```python
from build123d import *

# Parameters (mm, degrees)
BOSS_EXTRUDE1_DEPTH = 10
BOSS_EXTRUDE2_START = -5
SKETCH1_4_R         = 1.1
BOSS_EXTRUDE2_DEPTH = 5
FILLET1_R           = 3
SKETCH4_W           = 7.2
SKETCH4_H           = 7.2
CUT_EXTRUDE1_DEPTH  = 10
CIRPATTERN1_COUNT   = 3


with BuildPart() as part:
    # Sketch1 → Boss-Extrude1 (new body)
    with BuildSketch(Plane.XY):
        with BuildLine():
            ThreePointArc((-5.777817459, -11.645463727), (-3.344718433, -12.562358799), (-0.777817459, -12.976709907))
            Line((-0.777817459, -12.976709907), (-0.777817459, -0.777817459))
            ThreePointArc((-0.777817459, -0.777817459), (-0.420951776, 1.016267486), (1.1, 0))
            ThreePointArc((1.1, 0), (1.016267486, -0.420951776), (0.777817459, -0.777817459))
            Line((0.777817459, -0.777817459), (0.777817459, -12.976709907))
            ThreePointArc((0.777817459, -12.976709907), (3.344718433, -12.562358799), (5.777817459, -11.645463727))
            ThreePointArc((5.777817459, -11.645463727), (11.047887286, -6.851582774), (13, 0))
            ThreePointArc((13, 0), (-6.851582774, 11.047887286), (-5.777817459, -11.645463727))
        make_face()
        with BuildLine():
            Line((-5.777817459, -20.777817459), (-0.777817459, -20.777817459))
            Line((-0.777817459, -20.777817459), (-0.777817459, -12.976709907))
            ThreePointArc((-0.777817459, -12.976709907), (-3.344718433, -12.562358799), (-5.777817459, -11.645463727))
            Line((-5.777817459, -11.645463727), (-5.777817459, -20.777817459))
        make_face()
        with BuildLine():
            ThreePointArc((5.777817459, -11.645463727), (3.344718433, -12.562358799), (0.777817459, -12.976709907))
            Line((0.777817459, -12.976709907), (0.777817459, -20.777817459))
            Line((0.777817459, -20.777817459), (5.777817459, -20.777817459))
            Line((5.777817459, -20.777817459), (5.777817459, -11.645463727))
        make_face()
    extrude(amount=BOSS_EXTRUDE1_DEPTH)

    # Sketch1_4 → Boss-Extrude2 (add)
    with BuildSketch(Plane.XY.offset(BOSS_EXTRUDE2_START)):
        with BuildLine():
            ThreePointArc((-5.777817459, -11.645463727), (-3.344718433, -12.562358799), (-0.777817459, -12.976709907))
            Line((-0.777817459, -12.976709907), (-0.777817459, -0.777817459))
            ThreePointArc((-0.777817459, -0.777817459), (-0.420951776, 1.016267486), (1.1, 0))
            ThreePointArc((1.1, 0), (1.016267486, -0.420951776), (0.777817459, -0.777817459))
            Line((0.777817459, -0.777817459), (0.777817459, -12.976709907))
            ThreePointArc((0.777817459, -12.976709907), (3.344718433, -12.562358799), (5.777817459, -11.645463727))
            ThreePointArc((5.777817459, -11.645463727), (11.047887286, -6.851582774), (13, 0))
            ThreePointArc((13, 0), (-6.851582774, 11.047887286), (-5.777817459, -11.645463727))
        make_face()
        with BuildLine():
            Line((-0.777817459, -0.777817459), (-0.777817459, -12.976709907))
            ThreePointArc((-0.777817459, -12.976709907), (0, -13), (0.777817459, -12.976709907))
            Line((0.777817459, -12.976709907), (0.777817459, -0.777817459))
            ThreePointArc((0.777817459, -0.777817459), (0, -1.1), (-0.777817459, -0.777817459))
        make_face()
        with BuildLine():
            ThreePointArc((-5.777817459, -11.645463727), (-3.344718433, -12.562358799), (-0.777817459, -12.976709907))
            Line((-0.777817459, -12.976709907), (-0.777817459, -0.777817459))
            ThreePointArc((-0.777817459, -0.777817459), (-0.420951776, 1.016267486), (1.1, 0))
            ThreePointArc((1.1, 0), (1.016267486, -0.420951776), (0.777817459, -0.777817459))
            Line((0.777817459, -0.777817459), (0.777817459, -12.976709907))
            ThreePointArc((0.777817459, -12.976709907), (3.344718433, -12.562358799), (5.777817459, -11.645463727))
            ThreePointArc((5.777817459, -11.645463727), (11.047887286, -6.851582774), (13, 0))
            ThreePointArc((13, 0), (-6.851582774, 11.047887286), (-5.777817459, -11.645463727))
        make_face()
        with BuildLine():
            Line((-0.777817459, -0.777817459), (-0.777817459, -12.976709907))
            ThreePointArc((-0.777817459, -12.976709907), (0, -13), (0.777817459, -12.976709907))
            Line((0.777817459, -12.976709907), (0.777817459, -0.777817459))
            ThreePointArc((0.777817459, -0.777817459), (0, -1.1), (-0.777817459, -0.777817459))
        make_face()
        Circle(SKETCH1_4_R)
    extrude(amount=BOSS_EXTRUDE2_DEPTH)

    # Fillet1
    fillet1_edges = [part.edges().sort_by_distance(p)[0] for p in [
        (5.777817459, 11.645463727, -5),
    ]]
    fillet(fillet1_edges, radius=FILLET1_R)

    # Sketch4 → Cut-Extrude1 (cut)
    with BuildSketch(Plane(origin=(-11.286443879, -6.451305765, 0), x_dir=(0.499999999999998, -0.8660254037844398, 0), z_dir=(0.8660254037844398, 0.499999999999998, 0))):
        with Locations((0.056227259, -2.4)):
            Rectangle(SKETCH4_W, SKETCH4_H)
    cut_extrude1 = extrude(amount=CUT_EXTRUDE1_DEPTH, mode=Mode.SUBTRACT)

    # CirPattern1: Cut-Extrude1 ×3 about axis
    cirpattern1_axis = Axis((0, 0, 0), (0, 0, 1))
    for i in range(1, CIRPATTERN1_COUNT):
        add(cut_extrude1.rotate(cirpattern1_axis, i * 360 / CIRPATTERN1_COUNT), mode=Mode.SUBTRACT)


solid = part.part
```
Input: part model. Units: mm. Frame: model coordinates. A direction names the side the tool comes from. Give positions to 0.01 mm unless a question says otherwise; leave off trailing zeros. Order: outer loops, then holes, each group sorted by start corner. A loop starts at its lowest first (then second) coordinate and runs counter-clockwise, first axis right, second up. Notation, with made-up numbers: M 52.25,54.25 L 87.25,54.25 A30 cw 87.25,82.25 Z; hole C 80,45 d1. An arc over 180 degrees is marked long. Return JSON: item names as keys, results as strings.
1) Section query C-C on z = 6.5. Output: boundary loops of the cut face in (x, y).
Taken from the geometry:
{"outline": "M -5.78,-20.78 L -0.78,-20.78 L -0.78,-0.78 A1.1 cw long 0.78,-0.78 L 0.78,-20.78 L 5.78,-20.78 L 5.78,-11.65 A13 ccw long -5.78,-11.65 Z"}
2) Section query B-B on z = 3.5. Output: boundary loops of the cut face in (x, y).
Taken from the geometry:
{"outline": "M -12.62,-3.13 L -4.4,1.62 L -0.8,-4.62 L -9.02,-9.36 A13 ccw -5.78,-11.65 L -5.78,-20.78 L -0.78,-20.78 L -0.78,-0.78 A1.1 cw long 0.78,-0.78 L 0.78,-20.78 L 5.78,-20.78 L 5.78,-11.65 A13 ccw 9.02,-9.36 L 0.8,-4.62 L 4.4,1.62 L 12.62,-3.13 A13 ccw 3.6,12.49 L 3.6,3 L -3.6,3 L -3.6,12.49 A13 ccw Z"}
3) Line query: L1, parallel to Z at x = 3, y = 8.5; L2, parallel to Y at x = 0, z = 7.25; L3, parallel to X at y = -13, z = 0.75. Output: solid intervals per line, ascending. Write a range as [from, to].
Taken from the geometry:
{"L1": "z = [-5, -1.2], [6, 10]", "L2": "y = [1.1, 13]", "L3": "x = [-5.78, -0.78], [0.78, 5.78]"}
4) Section query A-A on y = -18. Output: boundary loops of the cut face in (x, z).
Taken from the geometry:
{"outline": "M -5.78,0 L -0.78,0 L -0.78,10 L -5.78,10 Z; M 0.78,0 L 5.78,0 L 5.78,10 L 0.78,10 Z"}
5) Access query for faces 1 (the face through (-7, -4, 6)), 2 (the face through (-3.6, 8, 2)), 3 (the face through (-0.778, -11, 5)), 4 (the face through (-3, -20.778, 5)), 5 (the face through (-5.778, -16, 5)). Directions: +Z, -Z, +X, -X, +Y, -Y. A direction counts if a zero-diameter tool reaches every point of the face in a straight line with its end or side. Return the directions, or none.
Taken from the geometry:
{"face 1": "none", "face 2": "+Y", "face 3": "+Z, -Y", "face 4": "+Z, -Z, +X, -X, -Y", "face 5": "+Z, -Z, -X, -Y"}
6) Section query D-D on y = -2. Count the separate pieces of the cut face and the enclosed holes in it, and give its area (3 significant figures).
Taken from the geometry:
{"separate pieces": "1", "enclosed holes": "2", "area": "246 mm2"}
7) Contact query for flat-ended pins moving along their axis: pin 1 (3 mm diameter, centred on y = -8, z = 4, fed in from -X); pin 2 (1.8 mm diameter, centred on x = 0, y = 0, fed in from +Z); pin 3 (3 mm diameter, centred on x = 0, z = -3.5, fed in from -Y). Output: stop coordinate, or through.
Taken from the geometry:
{"pin 1": "stops at x = -9.02", "pin 2": "stops at z = 0", "pin 3": "stops at y = -13"}
8) Mould query, pull axis X, two halves, no side actions, for faces 6 (the face through (3, 0, 10)), 7 (the face through (7, -4, 6)), 8 (the face through (5.778, -16, 5)). Classes: released by +X, released by -X, zero draft, split by the parting line, or undercut.
Taken from the geometry:
{"face 6": "zero draft", "face 7": "undercut", "face 8": "released by +X"}
